Geometry check sheet. Reference: drawing and pictorial views, mm from the part's lowest x, y, z. A direction names the side the tool comes from. Give positions to 0.01 mm unless a question says otherwise; leave off trailing zeros. Write each loop counter-clockwise with the first axis right and the second up, starting at its lowest first coordinate (ties: lowest second). Pieces come first, ordered by that corner, then holes. Notation, with made-up numbers: M 63.25,80.5 L 74.25,80.5 A28 ccw 74.25,117.5 Z; hole C -14,89.5 d4. An arc over 180 degrees is marked long. One line per item, written item: value. Start each with the question number.
1. Scan lines: line 1 (Y direction, x = 18, z = 15.5); line 2 (Z direction, x = 33.5, y = 12); line 3 (X direction, y = 21, z = 9.75) (1 decimal). Record each from-to range of solid material in increasing order.
2. Release check for a two-part mould opening along X. For the marked faces 1, 2, 3 and 4 record: pulls with the +X half, pulls with the -X half, needs draft (parallel to the pull), parting line crosses it, or undercut.
3. Cross-section at A-A on x = 18. Record the cut outline in (y, z).
4. Gauge pin test, flat ends, axial feed: pin 1 (2 mm diameter, centred on y = 16, z = 7.5, fed in from +X); pin 2 (2 mm diameter, centred on x = 19, z = 7.5, fed in from -Y); pin 3 (10 mm diameter, centred on x = 22, z = 4.5, fed in from +Y). Record the tip position at first contact, or that the pin passes through.
5. Cross-section at C-C on y = 12. Record the cut outline in (x, z).
6. Cross-section at B-B on z = 4.25. Record the cut outline in (x, y).
7. Tool access check on the marked faces 5, 6, 7 and 8. Record the directions out of +Z, -Z, +X, -X, +Y, -Y that give a thin tool (end or side, any length) a straight path to the whole face; none if there is none.
8. Cross-section at D-D on x = 6.5. Record the cut outline in (y, z), then the cut area to 3 significant figures.
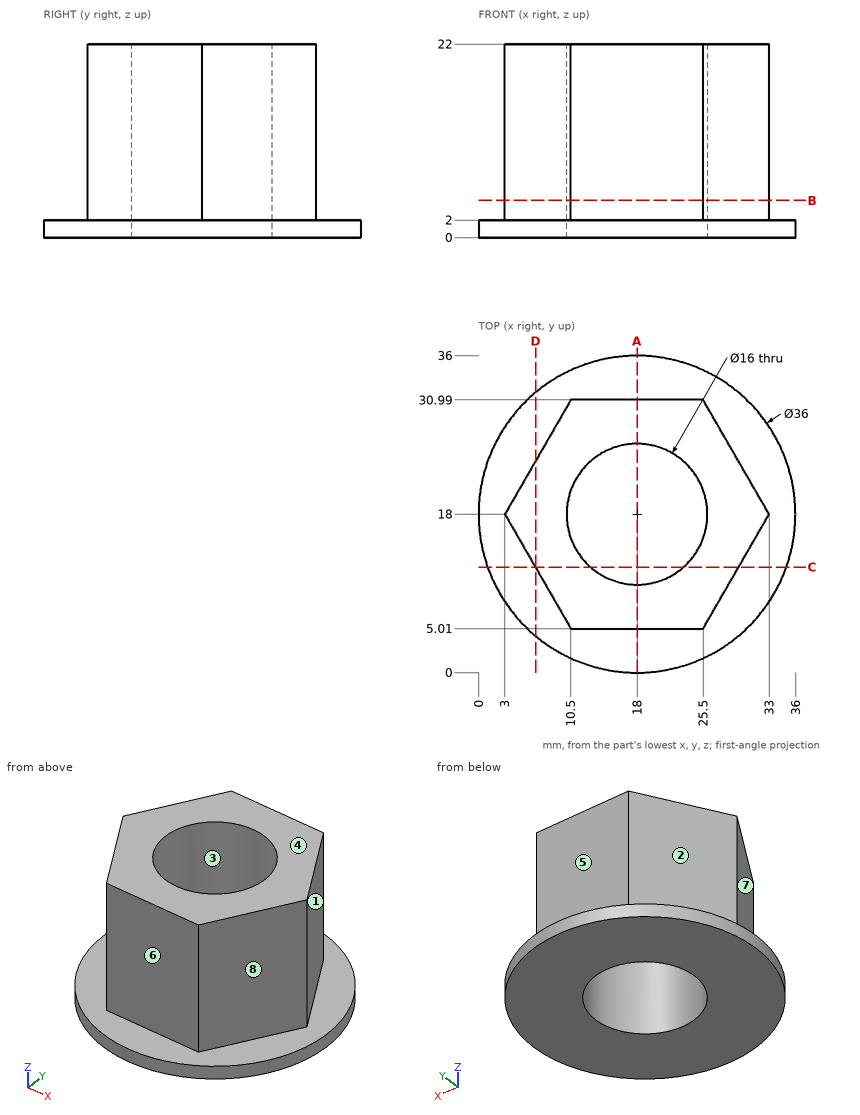
Report:
1. line 1: y = 5.01 to 10, 26 to 30.99
1. line 2: z = 0 to 2
1. line 3: x = 4.7 to 10.6, 25.4 to 31.3
2. face 1: pulls with the +X half
2. face 2: pulls with the -X half
2. face 3: undercut
2. face 4: needs draft
3. outline: M 0,0 L 10,0 L 10,22 L 5.01,22 L 5.01,2 L 0,2 Z; M 26,0 L 36,0 L 36,2 L 30.99,2 L 30.99,22 L 26,22 Z
4. pin 1: stops at x = 32.42
4. pin 2: stops at y = 5.01
4. pin 3: stops at y = 36
5. outline: M 1.03,0 L 12.71,0 L 12.71,22 L 6.46,22 L 6.46,2 L 1.03,2 Z; M 23.29,0 L 34.97,0 L 34.97,2 L 29.54,2 L 29.54,22 L 23.29,22 Z
6. outline: M 3,18 L 10.5,5.01 L 25.5,5.01 L 33,18 L 25.5,30.99 L 10.5,30.99 Z; hole C 18,18 d16
7. face 5: +Z, +X, -X, +Y
7. face 6: +Z, +X, -X, -Y
7. face 7: +Z, -X, -Y
7. face 8: +Z, +X, -Y
8. outline: M 4.15,0 L 31.85,0 L 31.85,2 L 24.06,2 L 24.06,22 L 11.94,22 L 11.94,2 L 4.15,2 Z
8. area: 298 mm^2
